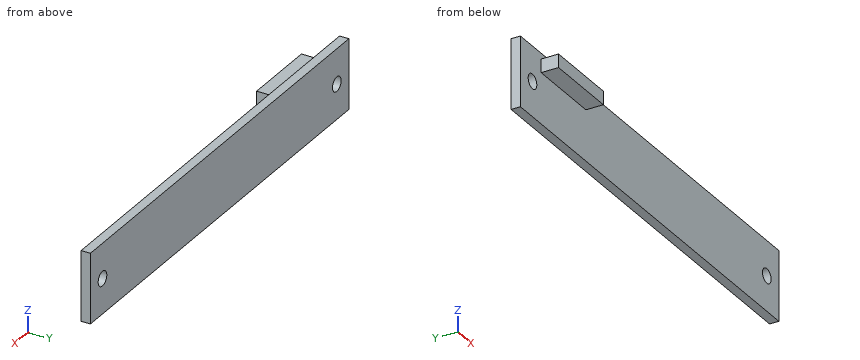
from build123d import *

# Parameters (mm, degrees)
SKETCH1_W           = 75
SKETCH1_H           = 12
PCB_DEPTH           = 1.6
SKETCH2_R           = 1.25
SCREW_HOLES_DEPTH   = 76.970783858
SKETCH3_W           = 13
SKETCH3_H           = 2.3
BOSS_EXTRUDE1_DEPTH = 3


with BuildPart() as part:
    # Sketch1 → pcb (new body)
    with BuildSketch(Plane(origin=(0, 0, 0), x_dir=(1, 0, 0), z_dir=(0, 1, 0))):
        with Locations((-37.5, 6)):
            Rectangle(SKETCH1_W, SKETCH1_H)
    extrude(amount=PCB_DEPTH)

    # Sketch2 → screw holes (cut, through all)
    with BuildSketch(Plane(origin=(0, 1.6, 0), x_dir=(1, 0, 0), z_dir=(0, 1, 0))):
        with Locations(Location((-71.5, 6, 0), (0, 0, 270))):
            Circle(SKETCH2_R)
        with Locations(Location((-3.5, 6, 0), (0, 0, 270))):
            Circle(SKETCH2_R)
    extrude(amount=-SCREW_HOLES_DEPTH, mode=Mode.SUBTRACT)

    # Sketch3 → Boss-Extrude1 (add)
    with BuildSketch(Plane.XZ):
        with Locations((-62.5, -2.15)):
            Rectangle(SKETCH3_W, SKETCH3_H)
    extrude(amount=BOSS_EXTRUDE1_DEPTH)


solid = part.part
Could you check a few things on this model? Use its own coordinates, in mm. Give positions to 0.01 mm unless a question says otherwise; leave off trailing zeros. Loops run counter-clockwise (first coordinate to the right, second up) from the corner with the lowest first, then second, coordinate; pieces in that order, holes last. Notation, with made-up numbers: (-5.75, 16.5) -> (12.25, 16.5) arc R12 ccw to (12.25, 35.5) -> close; hole circle Ø5 at (57, 25). An arc over 180 degrees is marked (long way). Return JSON: item names as keys, results as strings.
Item 1: If we section it at D-D on x = -62.5: List the corners of the cut face in (y, z) for me.
Geometry results:
{"outline": "(-3, -3.3) -> (0, -3.3) -> (0, -12) -> (1.6, -12) -> (1.6, 0) -> (0, 0) -> (0, -1) -> (-3, -1) -> close"}
Item 2: I'm going to push flat-ended pins straight in: pin 1 (1.8 mm diameter, centred on y = -2, z = -2.5, fed in from +X); pin 2 (1.5 mm diameter, centred on x = -3.5, z = -6, fed in from +Y); pin 3 (5 mm diameter, centred on x = -22, z = -2, fed in from -Y); pin 4 (2.5 mm diameter, centred on x = -60.5, y = -1.5, fed in from +Z). Where does each tip first touch, or does it pass through?
Geometry results:
{"pin 1": "stops at x = -56", "pin 2": "passes through", "pin 3": "stops at y = 0", "pin 4": "stops at z = -1"}
Item 3: If we section it at B-B on x = -71.5: List the corners of the cut face in (y, z) for me.
Geometry results:
{"outline": "(0, -12) -> (1.6, -12) -> (1.6, -7.25) -> (0, -7.25) -> close; (0, -4.75) -> (1.6, -4.75) -> (1.6, 0) -> (0, 0) -> close"}
Item 4: If we section it at A-A on z = -6: List the corners of the cut face in (x, y) for me, plus the area to 3 significant figures.
Geometry results:
{"outline": "(-75, 0) -> (-72.75, 0) -> (-72.75, 1.6) -> (-75, 1.6) -> close; (-70.25, 0) -> (-4.75, 0) -> (-4.75, 1.6) -> (-70.25, 1.6) -> close; (-2.25, 0) -> (0, 0) -> (0, 1.6) -> (-2.25, 1.6) -> close", "area": "112 mm²"}
Item 5: If we section it at C-C on z = -2: List the corners of the cut face in (x, y) for me, plus the area to 3 significant figures.
Geometry results:
{"outline": "(-75, 0) -> (-69, 0) -> (-69, -3) -> (-56, -3) -> (-56, 0) -> (0, 0) -> (0, 1.6) -> (-75, 1.6) -> close", "area": "159 mm²"}
Item 6: I need wall thicknesses on L1, parallel to X at y = 0.5, z = -6; L2, parallel to X at y = 0.2, z = -6.5; L3, parallel to Z at x = -71.5, y = 0.4. Which ranges of each line are inside material? Lowest first, please. Write a range as from..to.
Geometry results:
{"L1": "x = -75..-72.75, -70.25..-4.75, -2.25..0", "L2": "x = -75..-72.65, -70.35..-4.65, -2.35..0", "L3": "z = -12..-7.25, -4.75..0"}
